from build123d import *

# Parameters (mm, degrees)
EXTRUDE_1_DEPTH     = 60
FILLET_1_R          = 30
CUT_EXTRUDE_1_DEPTH = 147.1512713
SKETCH_4_R          = 10
EXTRUDE_3_DEPTH     = 12
FILLET_2_R          = 20
SKETCH_5_R          = 9
CUT_EXTRUDE_3_DEPTH = 15


with BuildPart() as part:
    # 스케치1 → 보스-돌출1 (new body)
    with BuildSketch(Plane.XY):
        Polygon((-22.843222842, 40.291179042), (43.149322352, -28.04610199), (43.149322352, -108.04610199), (58.149322352, -108.04610199), (58.149322352, -21.985708603), (-12.053125837, 50.711054599), align=None)
    extrude(amount=EXTRUDE_1_DEPTH)

    # 필렛1
    fillet_1_edges = [part.edges().sort_by_distance(p)[0] for p in [
        (-17.448174339, 45.50111682, 0),
        (-17.448174339, 45.50111682, 60),
    ]]
    fillet(fillet_1_edges, radius=FILLET_1_R - 0.0001)  # a hair under: the kernel refuses the full size

    # 스케치2 → 컷-돌출1 (cut, through all)
    with BuildSketch(Plane(origin=(19.103194466, 18.447740459, 0), x_dir=(0, 0, -1), z_dir=(0.7193398003386495, 0.694658370458999, 0))):
        with BuildLine():
            Line((-17, 14.851284643), (-17, -23.148715357))
            ThreePointArc((-17, -23.148715357), (-30, -36.148715357), (-43, -23.148715357))
            Line((-43, -23.148715357), (-43, 14.851284643))
            ThreePointArc((-43, 14.851284643), (-30, 27.851284643), (-17, 14.851284643))
        make_face()
    extrude(amount=-CUT_EXTRUDE_1_DEPTH, mode=Mode.SUBTRACT)

    # 스케치4 → 보스-돌출3 (add)
    with BuildSketch(Plane(origin=(0, 0, 0), x_dir=(-1, 0, 0), z_dir=(0, 0, -1))):
        with BuildLine():
            ThreePointArc((-121.787629996, -63.881157116), (-130.624090494, -38.115312537), (-108.674200792, -21.985708603))
            Line((-108.674200792, -21.985708603), (-58.149322352, -21.985708603))
            Line((-58.149322352, -21.985708603), (-58.149322352, -108.04610199))
            Line((-58.149322352, -108.04610199), (-121.787629996, -63.881157116))
        make_face()
        with Locations((-108.674200792, -44.985708603)):
            Circle(SKETCH_4_R, mode=Mode.SUBTRACT)
    extrude(amount=-EXTRUDE_3_DEPTH)

    # 필렛2
    fillet_2_edges = [part.edges().sort_by_distance(p)[0] for p in [
        (50.649322352, -108.04610199, 60),
    ]]
    fillet(fillet_2_edges, radius=FILLET_2_R)

    # 스케치5 → 컷-돌출3 (cut)
    with BuildSketch(Plane(origin=(58.149322352, 0, 0), x_dir=(0, 0, -1), z_dir=(1, 0, 0))):
        with Locations(Location((-40, -88.04610199, 0), (0, 0, 90))):
            Circle(SKETCH_5_R)
    extrude(amount=-CUT_EXTRUDE_3_DEPTH, mode=Mode.SUBTRACT)


solid = part.part
Work out the finished part from the listing and answer in its coordinate system (mm). A direction names the side the tool comes from. Round coordinates to 2 decimals unless told otherwise and drop trailing zeros. Write each loop counter-clockwise with the first axis right and the second up, starting at its lowest first coordinate (ties: lowest second). Pieces come first, ordered by that corner, then holes. Notation, with made-up numbers: (15, 16.25) -> (58, 16.25) arc R26 ccw to (58, 43.25) -> close; hole circle Ø1 at (62, 81.25). An arc over 180 degrees is marked (long way). Answer as CSV lines item,"result". Start each with the question number.
(1) The part is cut by section A-A, the plane z = 22.5. Give the vertices of the cut face in (x, y).
(2) The part is cut by section D-D, the plane y = -62. Give the vertices of the cut face in (x, z).
(3) Find the intervals of material crossed by probe 1 along Z at (x, y) = (72.5, -70); probe 2 along X at (y, z) = (-74, 18.5); probe 3 along X at (y, z) = (-48.5, 10.5), in increasing order.
(4) A tool of negligible diameter and unlimited length cuts with its end or side. For faces 1 (the flat face through (58.149, -66, 36)), 2 (the flat face through (44, -25, 60)), 3 (the flat face through (16, 11, 17)), from which of +Z, -Z, +X, -X, +Y, -Y can it reach the whole face along a straight path? Write none if from no direction.
(5) Each of these flat-tipped pins is pushed along its axis until it touches: pin 1 (3.5 mm diameter, centred on x = 71, z = 6.5, fed in from +Y); pin 2 (3 mm diameter, centred on y = -60, z = 20.5, fed in from +X); pin 3 (16 mm diameter, centred on x = 108.67, y = -44.99, fed in from -Z). Where does it stop, or does it pass through?
(6) The part is cut by section B-B, the plane x = 52.5. Give the vertices of the cut face in (y, z).
(7) The mould has two halves that part along Y. Classify faces 4 (the flat face through (51, -108.046, 20)), 5 (the flat face through (84, -21.986, 6)), 6 (the flat face through (43.149, -67, 30)), 7 (the cylindrical face through (50.75, -94.68, 46.08)): +Y half, -Y half, draft (parallel to the pull), parting line (faces both ways), or undercut.
(8) The part is cut by section C-C, the plane z = 33.5. Give the vertices of the cut face in (x, y), then the cut area to 3 significant figures.
Output values:
1,outline,"(-22.18, 39.61) -> (-9.38, 26.35) -> (1.41, 36.77) -> (-11.39, 50.03) -> close; (31.77, -16.26) -> (43.15, -28.05) -> (43.15, -108.05) -> (58.15, -108.05) -> (58.15, -21.99) -> (42.56, -5.84) -> close"
2,outline,"(43.15, 0) -> (124.15, 0) -> (124.15, 12) -> (58.15, 12) -> (58.15, 60) -> (43.15, 60) -> close"
3,probe 1,"z = 0 to 12"
3,probe 2,"x = 43.15 to 58.15"
3,probe 3,"x = 43.15 to 99.31, 118.04 to 131.4"
4,face 1,"+Z, +X, +Y, -Y"
4,face 2,"+Z, +X, -X, +Y, -Y"
4,face 3,"none"
5,pin 1,"stops at y = -21.99"
5,pin 2,"stops at x = 58.15"
5,pin 3,"passes through"
6,outline,"(-108.05, 0) -> (-16.14, 0) -> (-16.14, 60) -> (-88.05, 60) arc R20 ccw to (-108.05, 40) -> close; hole circle Ø18 at (-88.05, 40)"
7,face 4,"-Y half"
7,face 5,"+Y half"
7,face 6,"draft"
7,face 7,"undercut"
8,outline,"(-22.7, 40.14) -> (-10.7, 27.72) -> (0.09, 38.14) -> (-11.91, 50.56) -> close; (33.09, -17.63) -> (43.15, -28.05) -> (43.15, -81.82) -> (58.15, -81.82) -> (58.15, -21.99) -> (43.88, -7.21) -> close; (43.15, -108.05) -> (58.15, -108.05) -> (58.15, -94.27) -> (43.15, -94.27) -> close"
8,area,"1,580 mm²"
